Source: CAD feature listing. Evaluate the final solid. Frame: model axes, mm. Face numbers are marked on the shaded views. Give positions to 0.01 mm unless a question says otherwise; leave off trailing zeros. Write each question's results on one line, items separated by ' | '. Start each with the question number.
(1) Pull-direction query (Z, two-part tool) for the marked faces 1 and 2; classes: pulls with the +Z half, pulls with the -Z half, needs draft (parallel to the pull), parting line crosses it, or undercut.
(2) Material intervals for line 1 along Y through (x, z) = (35, 8.75); line 2 along X through (y, z) = (134, 9.25); line 3 along Y through (x, z) = (0, 13.15), sorted ascending. Write a range as [from, to].
(3) Contact query for flat-ended pins moving along their axis: pin 1 (5 mm diameter, centred on x = 3.5, y = -110, fed in from -Z); pin 2 (3 mm diameter, centred on x = 72, y = -66.5, fed in from +Z). Output: stop coordinate, or through.
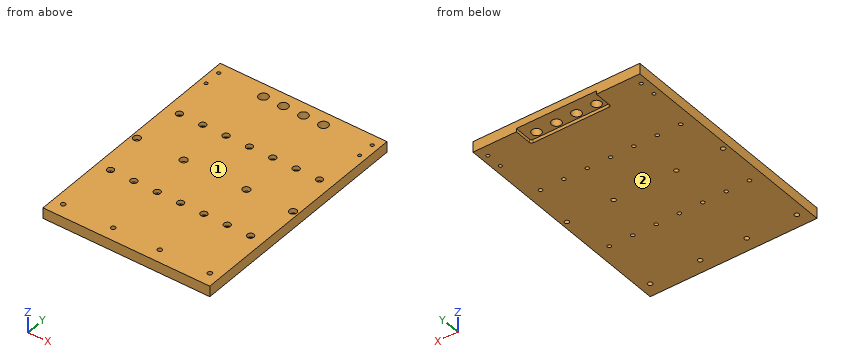
from build123d import *

# Parameters (mm, degrees)
SKETCH_1_W                  = 250
SKETCH_1_H                  = 350
EXTRUDE_1_DEPTH             = 16
HOLE_WIZARD_0_D             = 5.5
HOLE_WIZARD_0_DEPTH         = 22.25
HOLE_WIZARD_0_CBORE_D       = 10
HOLE_WIZARD_0_CBORE_DEPTH   = 5.7
HOLE_WIZARD_0_TIP           = 1.652366702
HOLE_WIZARD_0_2_D           = 6.6
HOLE_WIZARD_0_2_DEPTH       = 16
HOLE_WIZARD_0_2_CBORE_D     = 11
HOLE_WIZARD_0_2_CBORE_DEPTH = 6.8
MM_1_D                      = 6.8
MM_1_DEPTH                  = 22.25
MM_1_TIP                    = 2.042926105
HOLE_WIZARD_M6_1_D          = 5
HOLE_WIZARD_M6_1_DEPTH      = 20
HOLE_WIZARD_M6_1_TIP        = 1.502151548
MM_2_D                      = 14
MM_2_DEPTH                  = 15
MM_2_TIP                    = 4.206024333
SKETCH_12_W                 = 120
SKETCH_12_H                 = 29
CUT_EXTRUDE_1_DEPTH         = 5
FILLET_1_R                  = 3


with BuildPart() as part:
    # 草图1 → 凸台-拉伸1 (new body)
    with BuildSketch(Plane.XY):
        Rectangle(SKETCH_1_W, SKETCH_1_H)
    extrude(amount=EXTRUDE_1_DEPTH)

    # Hole Wizard 0
    with Locations(Plane(origin=(-70, 68, 16), x_dir=(1, 0, 0), z_dir=(0, 0, 1))):
        with Locations((0, 0), (35, 0), (70, 0), (105, 0), (140, 0), (-35, 0), (175, 0), (-35, -136), (0, -136), (35, -136), (70, -136), (105, -136), (140, -136), (175, -136)):
            CounterBoreHole(HOLE_WIZARD_0_D / 2, HOLE_WIZARD_0_CBORE_D / 2, HOLE_WIZARD_0_CBORE_DEPTH, depth=HOLE_WIZARD_0_DEPTH)
            with Locations((0, 0, -(HOLE_WIZARD_0_DEPTH + HOLE_WIZARD_0_TIP / 2))):  # 118° drill point
                Cone(0, HOLE_WIZARD_0_D / 2, HOLE_WIZARD_0_TIP, mode=Mode.SUBTRACT)

    # Hole Wizard 0 2
    with Locations(Plane(origin=(-47, 0, 16), x_dir=(1, 0, 0), z_dir=(0, 0, 1))):
        with Locations((0, 0), (94, 0), (-70, 0), (164, 0)):
            CounterBoreHole(HOLE_WIZARD_0_2_D / 2, HOLE_WIZARD_0_2_CBORE_D / 2, HOLE_WIZARD_0_2_CBORE_DEPTH, depth=HOLE_WIZARD_0_2_DEPTH)

    # 大小mm 暗销孔1
    with Locations(Plane(origin=(-110, -155, 16), x_dir=(1, 0, 0), z_dir=(0, 0, 1))):
        with Locations((0, 0), (75, 0), (145, 0), (220, 0)):
            Hole(MM_1_D / 2, depth=MM_1_DEPTH)
            with Locations((0, 0, -(MM_1_DEPTH + MM_1_TIP / 2))):  # 118° drill point
                Cone(0, MM_1_D / 2, MM_1_TIP, mode=Mode.SUBTRACT)

    # M6 螺纹孔1
    with Locations(Plane(origin=(-115, 159, 16), x_dir=(1, 0, 0), z_dir=(0, 0, 1))):
        with Locations((0, 0), (0, -25), (230, 0), (230, -25)):
            Hole(HOLE_WIZARD_M6_1_D / 2, depth=HOLE_WIZARD_M6_1_DEPTH)
            with Locations((0, 0, -(HOLE_WIZARD_M6_1_DEPTH + HOLE_WIZARD_M6_1_TIP / 2))):  # 118° drill point
                Cone(0, HOLE_WIZARD_M6_1_D / 2, HOLE_WIZARD_M6_1_TIP, mode=Mode.SUBTRACT)

    # 大小mm 暗销槽口2
    with Locations(Plane(origin=(-45, 155, 16), x_dir=(1, 0, 0), z_dir=(0, 0, 1))):
        with Locations((0, 0), (30, 0), (60, 0), (90, 0)):
            Hole(MM_2_D / 2, depth=MM_2_DEPTH)
            with Locations((0, 0, -(MM_2_DEPTH + MM_2_TIP / 2))):  # 118° drill point
                Cone(0, MM_2_D / 2, MM_2_TIP, mode=Mode.SUBTRACT)

    # 草图12 → 切除-拉伸1 (cut)
    with BuildSketch(Plane(origin=(0, 0, 0), x_dir=(-1, 0, 0), z_dir=(0, 0, -1))):
        with Locations((0, 160.5)):
            Rectangle(SKETCH_12_W, SKETCH_12_H)
    extrude(amount=-CUT_EXTRUDE_1_DEPTH, mode=Mode.SUBTRACT)

    # 圆角1
    fillet_1_edges = [part.edges().sort_by_distance(p)[0] for p in [
        (60, 146, 2.5),
        (-60, 146, 2.5),
    ]]
    fillet(fillet_1_edges, radius=FILLET_1_R)


solid = part.part
Ans:
1) face 1: pulls with the +Z half | face 2: pulls with the -Z half
2) line 1: [-175, -158.4], [-151.6, -70.75], [-65.25, 65.25], [70.75, 175] | line 2: [-125, -117.5], [-112.5, 112.5], [117.5, 125] | line 3: [-175, -73], [-63, 63], [73, 175]
3) pin 1: z = 0 | pin 2: z = 10.3
